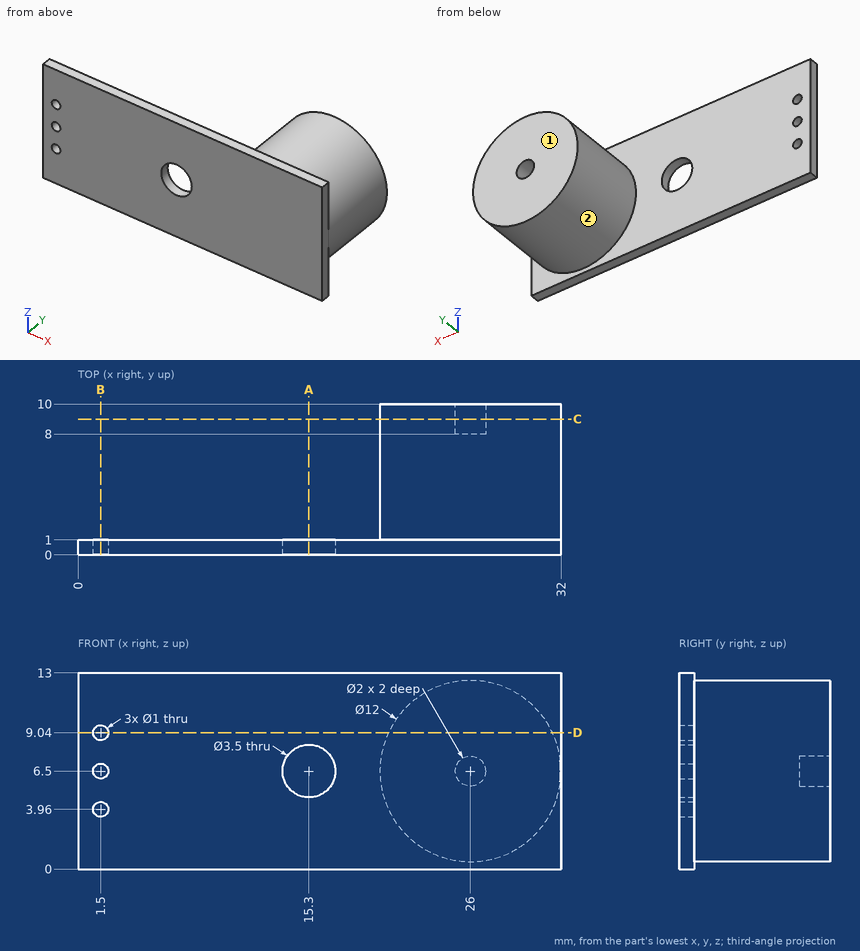
Design review of the part shown in the three views and the two pictorial views. Dimensions are in mm from the part's minimum x, y and z. A direction names the side the tool comes from. Round coordinates to 2 decimals unless told otherwise and drop trailing zeros. Write each loop counter-clockwise with the first axis right and the second up, starting at its lowest first coordinate (ties: lowest second). Pieces come first, ordered by that corner, then holes. Notation, with made-up numbers: (2, 71.25) -> (42, 71.25) arc R28 ccw to (42, 110.25) -> close; hole circle Ø1 at (63.5, -11). An arc over 180 degrees is marked (long way). Write item = value, one per line. Start each with the question number.
1) Take a section at D-D, the plane z = 9.04. State the section outline as (x, y) points, plus the area to 3 significant figures.
2) Clearance check with flat-ended pins moving along their axes: pin 1 (6.5 mm diameter, centred on x = 9, z = 6, fed in from +Y); pin 2 (2 mm diameter, centred on x = 20, y = 4.5, fed in from -Z); pin 3 (1 mm diameter, centred on x = 26, z = 6.5, fed in from +Y). State where each tip first meets the part, or that it passes through.
3) Wall thickness on probe 1 along X at (y, z) = (0.5, 6.5); probe 2 along Z at (x, y) = (1.5, 0.4); probe 3 along X at (y, z) = (0.75, 3.96): over which ranges is each line inside the solid? List them lowest first. Write a range as from..to.
4) Tool access review of the marked faces 1 and 2: name each direction out of +Z, -Z, +X, -X, +Y, -Y from which nothing blocks a thin tool from reaching the whole face with its end or side.
5) Take a section at A-A, the plane x = 15.3. State the section outline as (y, z) points.
6) Take a section at B-B, the plane x = 1.5. State the section outline as (y, z) points.
7) Take a section at C-C, the plane y = 9. State the section outline as (x, z) points, plus the area to 3 significant figures.
Results list:
q1.outline = (0, 0) -> (1, 0) -> (1, 1) -> (0, 1) -> close; (2, 0) -> (32, 0) -> (32, 1) -> (31.44, 1) -> (31.44, 10) -> (20.56, 10) -> (20.56, 1) -> (2, 1) -> close
q1.area = 129 mm²
q2.pin_1 = 1
q2.pin_2 = 3.18
q2.pin_3 = 8
q3.probe_1 = 0..1, 2..13.55, 17.05..32
q3.probe_2 = 0..3.46, 4.46..6, 7..8.54, 9.54..13
q3.probe_3 = 0..1, 2..32
q4.face_1 = +Z, -Z, +X, -X, +Y
q4.face_2 = +Y
q5.outline = (0, 0) -> (1, 0) -> (1, 4.75) -> (0, 4.75) -> close; (0, 8.25) -> (1, 8.25) -> (1, 13) -> (0, 13) -> close
q6.outline = (0, 0) -> (1, 0) -> (1, 3.46) -> (0, 3.46) -> close; (0, 4.46) -> (1, 4.46) -> (1, 6) -> (0, 6) -> close; (0, 7) -> (1, 7) -> (1, 8.54) -> (0, 8.54) -> close; (0, 9.54) -> (1, 9.54) -> (1, 13) -> (0, 13) -> close
q7.outline = circle Ø12 at (26, 6.5); hole circle Ø2 at (26, 6.5)
q7.area = 110 mm²
